Design review of the part built by this model. Coordinates are the model's own, in mm. A direction names the side the tool comes from. Coordinates: 2 decimals unless noted, no trailing zeros. Loops run counter-clockwise (first coordinate to the right, second up) from the corner with the lowest first, then second, coordinate; pieces in that order, holes last. Notation, with made-up numbers: (14.5, -25) -> (64.5, -25) arc R7 ccw to (64.5, -17) -> close; hole circle Ø2 at (-36.5, -2.5). An arc over 180 degrees is marked (long way). Use one line per item in the form item = value. Start each with the question number.
1. For pin 1 (1.6 mm diameter, centred on y = -1, z = 0, fed in from -X); pin 2 (2.5 mm diameter, centred on x = 2.5, y = -4.5, fed in from -Z); pin 3 (1 mm diameter, centred on x = -0.745, y = -4.6, fed in from +Z); pin 4 (3 mm diameter, centred on x = 6.5, z = 3.5, fed in from +Y), all flat-tipped, find the tip position at first contact; note any pin that passes through.
2. Machinability: for faces 1 (the face through (2.9, -4.06, -5.01)), 2 (the face through (0, -4, -4)), 3 (the face through (-2.337, -5.638, 5.014)), 4 (the face through (5.4, -1, 0)), 5 (the face through (-0.827, -2.466, -5.014)), which of the approach directions +Z, -Z, +X, -X, +Y, -Y give a long, thin tool a straight path to every point of the face, cutting with its end or side? Answer none if there is none.
3. Consider section B-B (z = -5.5). State the section outline as (x, y) points (3 decimals).
4. Consider section C-C (x = 2). State the section outline as (y, z) points, then the cut area to 3 significant figures.
5. Consider section D-D (y = -2.25). State the section outline as (x, z) points, then the cut area to 3 significant figures.
6. Consider section A-A (y = -4.6). State how many separate pieces and enclosed holes the cut face has, then the cut area to 3 significant figures.
7. Wall thickness on line 1 (Z direction, x = 4.5, y = -3.5); line 2 (Z direction, x = -1.25, y = -3.25); line 3 (Y direction, x = 1.25, z = -0.5): over which ranges is each line inside the solid? List them lowest first. Write a range as from..to.
8. The part is to be moulded in two halves that separate along Z. For faces 6 (the face through (0, -4, 4)), 7 (the face through (2.9, -4.06, 5.01)), 8 (the face through (0, -4, 6)), 9 (the face through (2.43, -4, 2.81)), say which applies: released by +Z, released by -Z, zero draft, split by the parting line, or undercut.
from build123d import *

# Parameters (mm, degrees)
EXTRUDE_1_DEPTH      = 8
EXTRUDE_1_DEPTH_BACK = 8
SKETCH_1_W           = 5.4
SKETCH_1_H           = 2
SKETCH_3_R           = 1.9
SKETCH_3_R_2         = 0.8
EXTRUDE_2_DEPTH      = 2
SKETCH_5_R           = 1
EXTRUDE_3_DEPTH      = 2


with BuildPart() as part:
    # Sketch 1 → Extrude 1 (new, two sides: drawn at the far end of the back side and taken through both)
    with BuildSketch(Plane.XY.offset(-EXTRUDE_1_DEPTH_BACK)):
        with Locations((2.7, -1)):
            Rectangle(SKETCH_1_W, SKETCH_1_H)
    extrude(amount=EXTRUDE_1_DEPTH + EXTRUDE_1_DEPTH_BACK)

    # Sketch 3 → Extrude 2 (add)
    # profile 1 of 2: a face of its own
    with BuildSketch(Plane.XY.offset(6)):
        with Locations((-0.745, -4.6)):
            Circle(SKETCH_3_R)
        with Locations((-0.745, -4.6)):
            Circle(SKETCH_3_R_2, mode=Mode.SUBTRACT)
    # profile 2 of 2: a face of its own
    with BuildSketch(Plane.XY.offset(6)):
        with BuildLine():
            Line((5.4, -2), (0, -2))
            Line((0, -2), (-1.677229227, -2.944418933))
            ThreePointArc((-1.677229227, -2.944418933), (0.213844218, -2.959689735), (1.155, -4.6))
            ThreePointArc((1.155, -4.6), (0.973307817, -5.410813325), (0.462980792, -6.066554604))
            Line((0.462980792, -6.066554604), (5.4, -2))
        make_face()
    extrude_2 = extrude(amount=-EXTRUDE_2_DEPTH)

    # Sketch 5 → Extrude 3 (add)
    with BuildSketch(Plane.XY.offset(3.8)):
        with BuildLine():
            Line((7.077229227, -2.944418933), (5.4, -2))
            Line((5.4, -2), (0, -2))
            Line((0, -2), (4.937019208, -6.066554604))
            ThreePointArc((4.937019208, -6.066554604), (7.712144702, -5.674270675), (7.077229227, -2.944418933))
        make_face()
        with Locations((6.145, -4.6)):
            Circle(SKETCH_5_R, mode=Mode.SUBTRACT)
    extrude_3 = extrude(amount=-EXTRUDE_3_DEPTH)

    # Mirror 1: Extrude 2, Extrude 3 across plane
    add(extrude_2.mirror(Plane.XY))
    add(extrude_3.mirror(Plane.XY))


solid = part.part
Geometry check:
q1.pin_1 = 0
q1.pin_2 = -6
q1.pin_3 = through
q1.pin_4 = 0
q2.face_1 = -Z, +X, -Y
q2.face_2 = +X, -X, -Y
q2.face_3 = +Z, -Z
q2.face_4 = +Z, -Z, +X, +Y
q2.face_5 = +Z, -Z, -X, +Y
q3.outline = (-1.677, -2.944) arc R1.9 ccw (long way) to (0.463, -6.067) -> (5.4, -2) -> (5.4, 0) -> (0, 0) -> (0, -2) -> close; hole circle Ø1.6 at (-0.745, -4.6)
q4.outline = (-4.8, -6) -> (-2, -6) -> (-2, -8) -> (0, -8) -> (0, 8) -> (-2, 8) -> (-2, 6) -> (-4.8, 6) -> (-4.8, 4) -> (-2, 4) -> (-2, 3.8) -> (-3.65, 3.8) -> (-3.65, 1.8) -> (-2, 1.8) -> (-2, -1.8) -> (-3.65, -1.8) -> (-3.65, -3.8) -> (-2, -3.8) -> (-2, -4) -> (-4.8, -4) -> close
q4.area = 49.8 mm²
q5.outline = (-0.44, -6) -> (5.1, -6) -> (5.1, -4) -> (-0.44, -4) -> close; (-0.44, 4) -> (5.1, 4) -> (5.1, 6) -> (-0.44, 6) -> close; (0.3, -3.8) -> (5.84, -3.8) -> (5.84, -1.8) -> (0.3, -1.8) -> close; (0.3, 1.8) -> (5.84, 1.8) -> (5.84, 3.8) -> (0.3, 3.8) -> close
q5.area = 44.3 mm²
q6.separate_pieces = 8
q6.enclosed_holes = 0
q6.area = 24.7 mm²
q7.line_1 = -3.8..-1.8, 1.8..3.8
q7.line_2 = -6..-4, 4..6
q7.line_3 = -2..0
q8.face_6 = undercut
q8.face_7 = zero draft
q8.face_8 = released by +Z
q8.face_9 = undercut
